Model file for the job. Use its own axes, mm. Face numbers are marked on the shaded views. Round coordinates to 2 decimals unless told otherwise and drop trailing zeros. Order: outer loops, then holes, each group sorted by start corner. A loop starts at its lowest first (then second) coordinate and runs counter-clockwise, first axis right, second up. Notation, with made-up numbers: M 84.5,74 L 129.5,74 A26 ccw 129.5,97 Z; hole C 1.5,42.25 d7. An arc over 180 degrees is marked long. Return JSON: item names as keys, results as strings. Group by question number.
Item 1: Slice it at C-C on y = -10. Write the cut outline in (x, z), then the cut area to 3 significant figures.
Item 2: Slice it at B-B on x = -2.35. Give the number of separate pieces and of enclosed holes in the cut face, then the cut area to 3 significant figures.
Item 3: Slice it at D-D on z = 20.5. Write the cut outline in (x, y).
Item 4: Pull direction Z, two halves, no side cores. Call the marked faces 1 and 2: pulls with the +Z half, pulls with the -Z half, needs draft (parallel to the pull), parting line crosses it, or undercut.
Item 5: Pin check, flat tip, straight feed: pin 1 Ø1.5 at (x, z) = (-2, 14.5) entering from -Y. Stop position of the tip, or through.
Item 6: Probe line 1 along Y through (x, z) = (-2.6, 13); line 2 along Y through (x, z) = (-2.15, 6.2); line 3 along Z through (x, y) = (-0.9, -10). List the from-to ranges inside material, lowest first.
Item 7: Slice it at A-A on z = 13.1. Write the cut outline in (x, y).
from build123d import *

# Parameters (mm, degrees)
ESQUISSE1_R        = 1.5
BOSS_EXTRU_1_DEPTH = 3


with BuildPart() as part:
    # Esquisse1 → Boss.-Extru.1 (new body)
    with BuildSketch(Plane(origin=(-3, 0, 0), x_dir=(0, -1, 0), z_dir=(-1, 0, 0))):
        Polygon((35, 27.2), (0, 27.2), (0, -1), (35, -1), (35, 3), (32, 3), (32, 23.2), (35, 23.2), align=None)
        with Locations(Location((5, 6.2, 0), (0, 0, 180))):
            Circle(ESQUISSE1_R, mode=Mode.SUBTRACT)
        with Locations(Location((10, 8, 0), (0, 0, 180))):
            Circle(ESQUISSE1_R, mode=Mode.SUBTRACT)
        with Locations(Location((15, 20, 0), (0, 0, 180))):
            Circle(ESQUISSE1_R, mode=Mode.SUBTRACT)
        with Locations(Location((5, 20, 0), (0, 0, 180))):
            Circle(ESQUISSE1_R, mode=Mode.SUBTRACT)
        with Locations(Location((15, 6.2, 0), (0, 0, 180))):
            Circle(ESQUISSE1_R, mode=Mode.SUBTRACT)
        with Locations(Location((10, 13.1, 0), (0, 0, 180))):
            Circle(ESQUISSE1_R, mode=Mode.SUBTRACT)
        with Locations(Location((10, 3, 0), (0, 0, 180))):
            Circle(ESQUISSE1_R, mode=Mode.SUBTRACT)
        with Locations(Location((5, 13.1, 0), (0, 0, 180))):
            Circle(ESQUISSE1_R, mode=Mode.SUBTRACT)
        with Locations(Location((15, 13.1, 0), (0, 0, 180))):
            Circle(ESQUISSE1_R, mode=Mode.SUBTRACT)
        with Locations(Location((9.99998284, 23.2, 0), (0, 0, 180))):
            Circle(ESQUISSE1_R, mode=Mode.SUBTRACT)
        with Locations(Location((9.99998284, 18.2, 0), (0, 0, 180))):
            Circle(ESQUISSE1_R, mode=Mode.SUBTRACT)
    extrude(amount=-BOSS_EXTRU_1_DEPTH)


solid = part.part
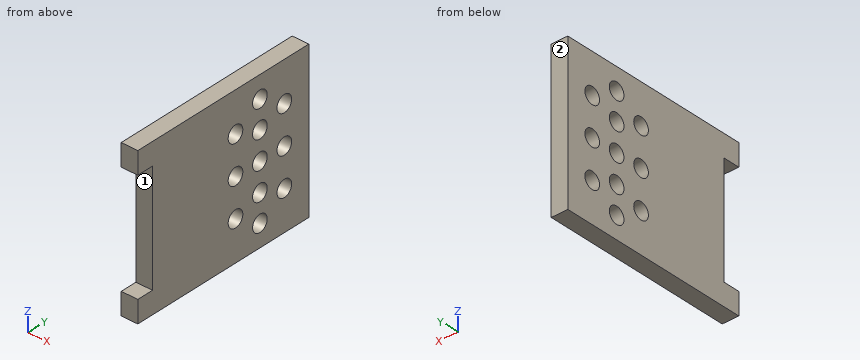
Output values:
{
 "1": {"outline": "M -3,-1 L 0,-1 L 0,1.5 L -3,1.5 Z; M -3,4.5 L 0,4.5 L 0,6.5 L -3,6.5 Z; M -3,9.5 L 0,9.5 L 0,11.6 L -3,11.6 Z; M -3,14.6 L 0,14.6 L 0,16.7 L -3,16.7 Z; M -3,19.7 L 0,19.7 L 0,21.7 L -3,21.7 Z; M -3,24.7 L 0,24.7 L 0,27.2 L -3,27.2 Z", "area": "39.6 mm²"},
 "2": {"separate pieces": "1", "enclosed holes": "11", "area": "849 mm²"},
 "3": {"outline": "M -3,-32 L 0,-32 L 0,-16.41 L -3,-16.41 Z; M -3,-13.59 L 0,-13.59 L 0,-6.41 L -3,-6.41 Z; M -3,-3.59 L 0,-3.59 L 0,0 L -3,0 Z"},
 "4": {"face 1": "undercut", "face 2": "needs draft"},
 "5": {"pin 1": "y = -32"},
 "6": {"line 1": "-32 to -16.5, -13.5 to -11.5, -8.5 to -6.5, -3.5 to 0", "line 2": "-32 to -16.5, -13.5 to -6.5, -3.5 to 0", "line 3": "-1 to 1.5, 4.5 to 6.5, 9.5 to 11.6, 14.6 to 16.7, 19.7 to 21.7, 24.7 to 27.2"},
 "7": {"outline": "M -3,-32 L 0,-32 L 0,-16.5 L -3,-16.5 Z; M -3,-13.5 L 0,-13.5 L 0,-11.5 L -3,-11.5 Z; M -3,-8.5 L 0,-8.5 L 0,-6.5 L -3,-6.5 Z; M -3,-3.5 L 0,-3.5 L 0,0 L -3,0 Z"}
}
